Here's the drawing with two shaded views (mm, measured from the low corner). I have some questions. Round coordinates to 2 decimals unless told otherwise and drop trailing zeros. Loops run counter-clockwise (first coordinate to the right, second up) from the corner with the lowest first, then second, coordinate; pieces in that order, holes last. Notation, with made-up numbers: M -8.75,-30.5 L 46.25,-30.5 A20 ccw 46.25,-14.5 Z; hole C 86.25,12.5 d9. An arc over 180 degrees is marked long. Answer as a JSON object with one key per item and string values.
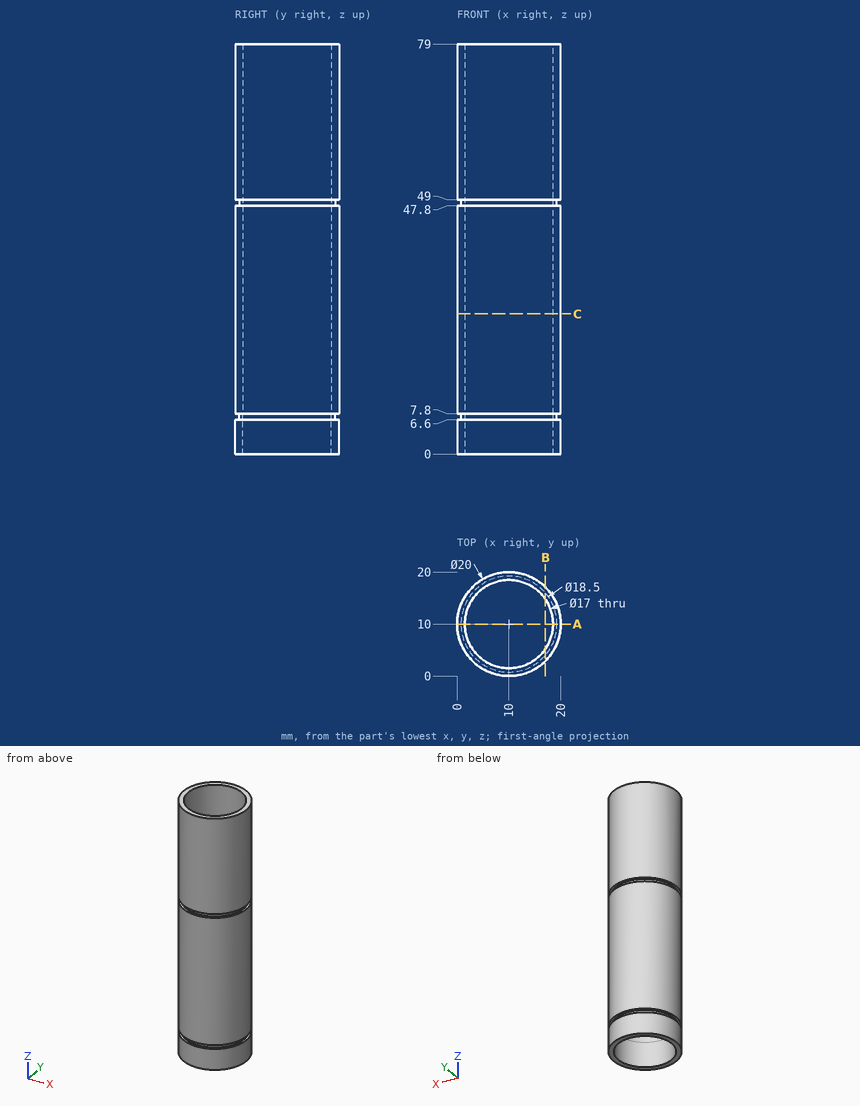
Item 1: I want a section at A-A on y = 10. List the corners of the cut face in (x, z) for me.
Solution:
{"outline": "M 0,0 L 1.5,0 L 1.5,79 L 0,79 L 0,49 L 0.75,49 L 0.75,47.8 L 0,47.8 L 0,7.8 L 0.75,7.8 L 0.75,6.6 L 0,6.6 Z; M 18.5,0 L 20,0 L 20,6.6 L 19.25,6.6 L 19.25,7.8 L 20,7.8 L 20,47.8 L 19.25,47.8 L 19.25,49 L 20,49 L 20,79 L 18.5,79 Z"}
Item 2: I want a section at B-B on x = 17. List the corners of the cut face in (y, z) for me, plus the area to 3 significant figures.
Solution:
{"outline": "M 2.86,0 L 5.18,0 L 5.18,79 L 2.86,79 L 2.86,49 L 3.95,49 L 3.95,47.8 L 2.86,47.8 L 2.86,7.8 L 3.95,7.8 L 3.95,6.6 L 2.86,6.6 Z; M 14.82,0 L 17.14,0 L 17.14,6.6 L 16.05,6.6 L 16.05,7.8 L 17.14,7.8 L 17.14,47.8 L 16.05,47.8 L 16.05,49 L 17.14,49 L 17.14,79 L 14.82,79 Z", "area": "361 mm2"}
Item 3: I want a section at C-C on z = 27. List the corners of the cut face in (x, y) for me, plus the area to 3 significant figures.
Solution:
{"outline": "C 10,10 d20; hole C 10,10 d17", "area": "87.2 mm2"}
Item 4: If I drill on L1, parallel to Y at x = 10, z = 1.75; L2, parallel to X at y = 4.5, z = 57, over which ranges is the centre line in solid material (lowest first)? Write a range as from..to.
Solution:
{"L1": "y = 0..1.5, 18.5..20", "L2": "x = 1.65..3.52, 16.48..18.35"}
Item 5: For P1, Ø12, axis at x = 16.5, z = 71, coming from the +Y side; P2, Ø5, axis at x = 16, z = 18.5, coming from the -Y side; P3, Ø6, axis at x = 10, y = 5.5, coming from the +Z side; P4, Ø3, axis at x = 12.5, z = 9.5, coming from the -Y side, each with a flat end and sliding along its axis, tell me the tip position at first contact or that it passes through.
Solution:
{"P1": "stops at y = 19.99", "P2": "stops at y = 0.63", "P3": "passes through", "P4": "stops at y = 0.05"}
